from build123d import *

# Parameters (mm, degrees)
EXTRUDE1_DEPTH      = 10.3
EXTRUDE1_DEPTH_BACK = 10.3
SKETCH1_W           = 11
SKETCH1_H           = 55
EXTRUDE2_DEPTH      = 6
SKETCH5_R           = 5.5
EXTRUDE4_DEPTH      = 69.744308855
SKETCH_1_R          = 2.8
CUT_EXTRUDE_1_DEPTH = 76.545350618
FILLET2_R           = 1.5
SKETCH_3_R          = 11.5
CUT_EXTRUDE_2_DEPTH = 8
SKETCH_4_R          = 1.3
CUT_EXTRUDE_3_DEPTH = 71.80805039
CHAMFER_1_SIZE      = 1


with BuildPart() as part:
    # Sketch1 → Extrude1 (new, two sides: drawn at the far end of the back side and taken through both)
    with BuildSketch(Plane(origin=(0, 0, 0), x_dir=(0, 0, -1), z_dir=(1, 0, 0)).offset(-EXTRUDE1_DEPTH_BACK)):
        with Locations((0, 37.8)):
            Rectangle(SKETCH1_W, SKETCH1_H)
    extrude(amount=EXTRUDE1_DEPTH + EXTRUDE1_DEPTH_BACK)

    # Sketch2 → Extrude2 (add)
    with BuildSketch(Plane(origin=(10.3, 0, 0), x_dir=(0, 0, -1), z_dir=(1, 0, 0))):
        with BuildLine():
            Line((-19.5, 10), (-19.5, -10))
            Line((-19.5, -10), (5.5, -10))
            Line((5.5, -10), (5.5, 17))
            Line((5.5, 17), (5.5, 65.3))
            Line((5.5, 65.3), (-5.5, 65.3))
            Line((-5.5, 65.3), (-5.5, 17))
            ThreePointArc((-5.5, 17), (-7.550252532, 12.050252532), (-12.5, 10))
            Line((-12.5, 10), (-19.5, 10))
        make_face()
    extrude2 = extrude(amount=EXTRUDE2_DEPTH)

    # Mirror2: Extrude2 across plane
    add(extrude2.mirror(Plane(origin=(0, 0, 0), x_dir=(0, 0, 1), z_dir=(1, 0, 0))))

    # Sketch5 → Extrude4 (cut, through all)
    with BuildSketch(Plane.XY.offset(5.5)):
        with Locations((0, 44)):
            Circle(SKETCH5_R)
    extrude(amount=-EXTRUDE4_DEPTH, mode=Mode.SUBTRACT)

    # Эскиз1 → Вырез-Вытянуть1 (cut, through all)
    with BuildSketch(Plane(origin=(16.3, 0, 0), x_dir=(0, 0, -1), z_dir=(1, 0, 0))):
        with Locations((-13, 0)):
            Circle(SKETCH_1_R)
        with Locations(Location((-1, 0, 0), (0, 0, 180))):
            Circle(SKETCH_1_R)
    extrude(amount=-CUT_EXTRUDE_1_DEPTH, mode=Mode.SUBTRACT)

    # Fillet2
    fillet2_edges = [part.edges().sort_by_distance(p)[0] for p in [
        (13.3, -10, 19.5),
        (13.3, -10, -5.5),
        (13.3, 10, 19.5),
        (-13.3, -10, -5.5),
        (-13.3, -10, 19.5),
        (-13.3, 10, 19.5),
        (0, 65.3, 5.5),
        (0, 65.3, -5.5),
    ]]
    fillet(fillet2_edges, radius=FILLET2_R)

    # Эскиз3 → Вырез-Вытянуть2 (cut)
    with BuildSketch(Plane.XY.offset(5.5)):
        with Locations((0, 44)):
            Circle(SKETCH_3_R)
    extrude(amount=-CUT_EXTRUDE_2_DEPTH, mode=Mode.SUBTRACT)

    # Эскиз4 → Вырез-Вытянуть3 (cut, through all)
    with BuildSketch(Plane.XY.offset(-2.5)):
        with Locations((0, 52.5)):
            Circle(SKETCH_4_R)
        with Locations((7.361215932, 39.75)):
            Circle(SKETCH_4_R)
        with Locations((-7.361215932, 39.75)):
            Circle(SKETCH_4_R)
    extrude(amount=-CUT_EXTRUDE_3_DEPTH, mode=Mode.SUBTRACT)

    # Фаска1
    # the kernel refuses this chamfer: 1 mm, written as the material it takes off along each edge
    with BuildSketch(Plane(origin=(0, 52.5, -5.5), x_dir=(1, 0, 0), z_dir=(0, -1, 0))) as chamfer_1_piece_1:
        Polygon((1.3 + CHAMFER_1_SIZE, 0), (1.3, CHAMFER_1_SIZE), (1.3, 0), align=None)
    revolve(axis=Axis((0, 52.5, -5.5), (0, 0, 1)), mode=Mode.SUBTRACT)
    with BuildSketch(Plane(origin=(7.361215932, 39.75, -5.5), x_dir=(1, 0, 0), z_dir=(0, -1, 0))) as chamfer_1_piece_2:
        Polygon((1.3 + CHAMFER_1_SIZE, 0), (1.3, CHAMFER_1_SIZE), (1.3, 0), align=None)
    revolve(axis=Axis((7.361215932, 39.75, -5.5), (0, 0, 1)), mode=Mode.SUBTRACT)
    with BuildSketch(Plane(origin=(-7.361215932, 39.75, -5.5), x_dir=(1, 0, 0), z_dir=(0, -1, 0))) as chamfer_1_piece_3:
        Polygon((1.3 + CHAMFER_1_SIZE, 0), (1.3, CHAMFER_1_SIZE), (1.3, 0), align=None)
    revolve(axis=Axis((-7.361215932, 39.75, -5.5), (0, 0, 1)), mode=Mode.SUBTRACT)
    with BuildSketch(Plane(origin=(0, 44, -5.5), x_dir=(1, 0, 0), z_dir=(0, -1, 0))) as chamfer_1_piece_4:
        Polygon((5.5 + CHAMFER_1_SIZE, 0), (5.5, CHAMFER_1_SIZE), (5.5, 0), align=None)
    revolve(axis=Axis((0, 44, -5.5), (0, 0, 1)), mode=Mode.SUBTRACT)


solid = part.part
Geometry: final body of the model. Coordinates: model frame, mm. A direction names the side the tool comes from. Round coordinates to 2 decimals unless told otherwise and drop trailing zeros. Loops run counter-clockwise (first coordinate to the right, second up) from the corner with the lowest first, then second, coordinate; pieces in that order, holes last. Notation, with made-up numbers: (2.25, 66) -> (47.25, 66) arc R25 ccw to (47.25, 101) -> close; hole circle Ø3 at (39.5, 70.5). An arc over 180 degrees is marked (long way). One line per question, with ' | ' between items. Start each with the question number.
1. Section A-A on y = 44. Output: boundary loops of the cut face in (x, z).
2. Contact query for flat-ended pins moving along their axis: pin 1 (9 mm diameter, centred on y = 0, z = 13, fed in from -X); pin 2 (5 mm diameter, centred on y = 0, z = 1, fed in from +X); pin 3 (10 mm diameter, centred on x = 2, y = 39.5, fed in from +Z); pin 4 (3 mm diameter, centred on x = 3.5, z = 3.5, fed in from -Y). Output: stop coordinate, or through.
3. Line query: line 1 along Y through (x, z) = (0, 2.75); line 2 along X through (y, z) = (-7, 7.5); line 3 along Y through (x, z) = (12.7, 13). Output: solid intervals per line, ascending. Write a range as [from, to].
4. Section D-D on x = -12.5. Output: boundary loops of the cut face in (y, z).
5. Section B-B on x = 0. Output: boundary loops of the cut face in (y, z), and give its area (3 significant figures).
6. Section C-C on z = 1.75. Output: boundary loops of the cut face in (x, y), and give its area (3 significant figures).
7. Mould query, pull axis Z, two halves, no side actions, for faces 1 (the face through (-13.34, -9.55, 19.07)), 2 (the face through (-13.3, -0.1, -1.8)), 3 (the face through (-10.3, 1, 7)). Classes: pulls with the +Z half, pulls with the -Z half, needs draft (parallel to the pull), parting line crosses it, or undercut.
8. Set-up query: faces 4 (the face through (0, 10.3, 0)), 5 (the face through (5, 47, -2.5)), 6 (the face through (13, 10, 15)). Return all of +Z, -Z, +X, -X, +Y, -Y with unobstructed straight access to the full face (end or side cutting, diameter ignored); none if empty.
Returned:
1) outline: (-16.3, -5.5) -> (-6.5, -5.5) -> (-5.5, -4.5) -> (-5.5, -2.5) -> (-11.5, -2.5) -> (-11.5, 5.5) -> (-16.3, 5.5) -> close; (5.5, -4.5) -> (6.5, -5.5) -> (16.3, -5.5) -> (16.3, 5.5) -> (11.5, 5.5) -> (11.5, -2.5) -> (5.5, -2.5) -> close
2) pin 1: stops at x = -16.3 | pin 2: passes through | pin 3: stops at z = -2.5 | pin 4: stops at y = 10.3
3) line 1: y = [10.3, 32.5], [55.5, 65.3] | line 2: x = [-16.3, -10.3], [10.3, 16.3] | line 3: y = [-10, -2.8], [2.8, 10]
4) outline: (-10, -4) arc R1.5 ccw to (-8.5, -5.5) -> (63.8, -5.5) arc R1.5 ccw to (65.3, -4) -> (65.3, 4) arc R1.5 ccw to (63.8, 5.5) -> (17, 5.5) arc R7 cw to (10, 12.5) -> (10, 18) arc R1.5 ccw to (8.5, 19.5) -> (-8.5, 19.5) arc R1.5 ccw to (-10, 18) -> close; hole circle Ø5.6 at (0, 1); hole circle Ø5.6 at (0, 13)
5) outline: (10.3, -5.5) -> (37.5, -5.5) -> (38.5, -4.5) -> (38.5, -2.5) -> (32.5, -2.5) -> (32.5, 5.5) -> (10.3, 5.5) -> close; (49.5, -4.5) -> (50.35, -5.35) -> (51.2, -4.5) -> (51.2, -2.5) -> (49.5, -2.5) -> close; (53.8, -4.5) -> (54.8, -5.5) -> (63.8, -5.5) arc R1.5 ccw to (65.3, -4) -> (65.3, 4) arc R1.5 ccw to (63.8, 5.5) -> (55.5, 5.5) -> (55.5, -2.5) -> (53.8, -2.5) -> close | area: 377 mm2
6) outline: (-16.3, -10) -> (-10.3, -10) -> (-10.3, -2.7) -> (-16.3, -2.7) -> close; (-16.3, 2.7) -> (-10.3, 2.7) -> (-10.3, 10.3) -> (10.3, 10.3) -> (10.3, 2.7) -> (16.3, 2.7) -> (16.3, 65.3) -> (-16.3, 65.3) -> close; (10.3, -10) -> (16.3, -10) -> (16.3, -2.7) -> (10.3, -2.7) -> close; hole circle Ø23 at (0, 44) | area: 1,560 mm2
7) face 1: pulls with the +Z half | face 2: undercut | face 3: needs draft
8) face 4: +Z, -Z, -Y | face 5: +Z | face 6: +Z, +X, -X, +Y
